Autodesk Inventor part; units mm, degrees
ref_plane "YZ Plane" through (0, 0, 0) normal (1, 0, 0) x (0, 1, 0)
ref_plane "XZ Plane" through (0, 0, 0) normal (0, 1, 0) x (-1, 0, 0)
ref_plane "XY Plane" through (0, 0, 0) normal (0, 0, 1) x (1, 0, 0)
sketch "Sketch1" plane through (0, 0, 0) normal (0, 1, 0) x (-1, 0, 0)
  line L0 (2, 0) -> (1, -1.7321)
  line L1 (1, -1.7321) -> (-1, -1.7321)
  line L2 (-1, -1.7321) -> (-2, 0)
  line L3 (-2, 0) -> (-1, 1.7321)
  line L4 (-1, 1.7321) -> (1, 1.7321)
  line L5 (1, 1.7321) -> (2, 0)
  circle A0 centre (0, 0) radius 1
extrude "Extrusion1" add sketch "Sketch1" along normal blind 5
sketch "Sketch2" plane through (0, 5, 0) normal (0, 1, 0) x (1, 0, 0)
  line L0 (-2, 0) -> (-1, 1.7321)
  line L1 (-1, 1.7321) -> (1, 1.7321)
  line L2 (1, 1.7321) -> (2, 0)
  line L3 (2, 0) -> (1, -1.7321)
  line L4 (1, -1.7321) -> (-1, -1.7321)
  line L5 (-1, -1.7321) -> (-2, 0)
  point P0 (0, 0)
  point P1 (0, 0)
extrude "Extrusion2" add sketch "Sketch2" against normal blind 0.1
sketch "Sketch3" plane through (0, 5, 0) normal (0, 1, 0) x (1, 0, 0)
  circle A0 centre (0, 0) radius 1
  dimension "d5" = 2
extrude "Extrusion3" add sketch "Sketch3" along normal blind 3.5
properties part number "Standoff"
Geometry: final body of the model. Coordinates: model frame, mm. A direction names the side the tool comes from. Coordinates: 2 decimals unless noted, no trailing zeros. Order: outer loops, then holes, each group sorted by start corner. A loop starts at its lowest first (then second) coordinate and runs counter-clockwise, first axis right, second up.
Item 1: Access query for faces 1 (the face through (1.51, 2.46, 0.85)), 2 (the face through (-1, 5, 1)). Directions: +Z, -Z, +X, -X, +Y, -Y. A direction counts if a zero-diameter tool reaches every point of the face in a straight line with its end or side. Return the directions, or none.
Answer:
face 1: +Z, +X, +Y, -Y
face 2: +Y
Item 2: Section query B-B (x = 0). Output: boundary loops of the cut face in (y, z), then the cut area to 3 significant figures.
Answer:
outline: (0, -1.73) - (5, -1.73) - (5, -1) - (8.5, -1) - (8.5, 1) - (5, 1) - (5, 1.73) - (0, 1.73) - (0, 1) - (4.9, 1) - (4.9, -1) - (0, -1) - close
area: 14.5 mm2
Item 3: Draft query along X for faces 3 (the face through (1.49, 2.46, -0.88)), 4 (the face through (0, 4.9, 0)), 5 (the face through (0, 2, 1)), 6 (the face through (0, 2, 1.732)). Return one class per face: released by +X, released by -X, zero draft, split by the parting line, or undercut.
Answer:
face 3: released by +X
face 4: undercut
face 5: undercut
face 6: zero draft
Item 4: Section query C-C (z = 0.4). Output: boundary loops of the cut face in (x, y).
Answer:
outline: (-1.77, 0) - (-0.92, 0) - (-0.92, 4.9) - (0.92, 4.9) - (0.92, 0) - (1.77, 0) - (1.77, 5) - (0.92, 5) - (0.92, 8.5) - (-0.92, 8.5) - (-0.92, 5) - (-1.77, 5) - close
Item 5: Section query D-D (y = 7.25). Output: boundary loops of the cut face in (x, z), then the cut area to 3 significant figures.
Answer:
outline: circle Ø2 at (0, 0)
area: 3.14 mm2
Item 6: Section query A-A (y = 0.5). Output: boundary loops of the cut face in (x, z), then the cut area to 3 significant figures.
Answer:
outline: (-2, 0) - (-1, -1.73) - (1, -1.73) - (2, 0) - (1, 1.73) - (-1, 1.73) - close; hole circle Ø2 at (0, 0)
area: 7.25 mm2
Item 7: Material intervals for line 1 along Z through (x, y) = (0, 3.5); line 2 along Y through (x, z) = (-0.95, -1); line 3 along X through (y, z) = (4.5, -0.3), sorted ascending.
Answer:
line 1: z = -1.73 to -1, 1 to 1.73
line 2: y = 0 to 5
line 3: x = -1.83 to -0.95, 0.95 to 1.83
